Could you check a few things on this model? Use its own coordinates, in mm. A direction names the side the tool comes from. Coordinates: 2 decimals unless noted, no trailing zeros. Write each loop counter-clockwise with the first axis right and the second up, starting at its lowest first coordinate (ties: lowest second). Pieces come first, ordered by that corner, then holes. Notation, with made-up numbers: M -24.5,64.5 L 12.5,64.5 A36 cw 12.5,99.5 Z; hole C 56,65.25 d10. An arc over 180 degrees is marked long. Write item = value, one per line.
```python
from build123d import *

# Parameters (mm, degrees)
SKETCH018_W  = 140
SKETCH018_H  = 10
PAD013_DEPTH = 2
SKETCH026_R  = 2.542055
PAD018_DEPTH = 1


with BuildPart() as part:
    # Sketch018 → Pad013 (new body)
    with BuildSketch(Plane.XY):
        with Locations((0, 20)):
            Rectangle(SKETCH018_W, SKETCH018_H)
    extrude(amount=-PAD013_DEPTH)

    # Sketch026 (on Face5 of Pad013) → Pad018 (join)
    with BuildSketch(Plane.XY):
        with Locations((-62.995332, 20.006431)):
            Circle(SKETCH026_R)
    pad018 = extrude(amount=PAD018_DEPTH)

    # Mirrored003: Pad018 across Sketch026 V_Axis
    add(pad018.mirror(Plane(origin=(0, 0, 0), x_dir=(0, 0, 1), z_dir=(1, 0, 0))))


solid = part.part
```
Item 1: For faces 3 (the face through (60.65, 19.03, 0.49)), 4 (the face through (-1, 20, -2)), which set-ups out of +Z, -Z, +X, -X, +Y, -Y let a thin tool reach every point of the face, with its end or its side?
Numbers:
face_3 = +Z
face_4 = -Z, +X, -X, +Y, -Y
Item 2: I'm going to push a flat-ended pin straight in: P1, Ø5, axis at x = 28, y = 19.5, coming from the +Z side. Where does the tip first touch, or does it pass through?
Numbers:
P1 = 0
Item 3: If we mould it in two halves opening along X, with no side actions, what happens to faces 1 (the face through (63, 20, 1)), 2 (the face through (-60.65, 19.03, 0.49))? For each: pulls with the +X half, pulls with the -X half, needs draft (parallel to the pull), parting line crosses it, or undercut.
Numbers:
face_1 = needs draft
face_2 = undercut
Item 4: If I drill on line 1 along X through (y, z) = (19.75, 0.75); line 2 along Z through (x, y) = (42, 18.5); line 3 along X through (y, z) = (18.5, 0.35), over which ranges is the centre line in solid material (lowest first)?
Numbers:
line_1 = -65.52 to -60.47, 60.47 to 65.52
line_2 = -2 to 0
line_3 = -65.04 to -60.95, 60.95 to 65.04
Item 5: Imagine slicing it at A-A (y = 16.25). Write out the boundary of the cut face in (x, z), and give its area (3 significant figures).
Numbers:
outline = M -70,-2 L 70,-2 L 70,0 L -70,0 Z
area = 280 mm²
Item 6: Imagine slicing it at B-B (x = 54). Write out the boundary of the cut face in (y, z).
Numbers:
outline = M 15,-2 L 25,-2 L 25,0 L 15,0 Z
